```python
from build123d import *

# Parameters (mm, degrees)
SKETCH1_W                                       = 40
SKETCH1_H                                       = 20
BOSS_EXTRUDE1_DEPTH                             = 35
SKETCH2_W                                       = 5
SKETCH2_H                                       = 20
BOSS_EXTRUDE2_DEPTH                             = 5
SKETCH3_R                                       = 3.75
BOSS_EXTRUDE3_DEPTH                             = 10
CSK_FOR_M2_FLAT_HEAD_MACHINE_SCREW2_D           = 2.4
CSK_FOR_M2_FLAT_HEAD_MACHINE_SCREW2_CSINK_D     = 4.4
CSK_FOR_M2_FLAT_HEAD_MACHINE_SCREW2_CSINK_ANGLE = 90


with BuildPart() as part:
    # Sketch1 → Boss-Extrude1 (new body)
    with BuildSketch(Plane(origin=(0, 0, 0), x_dir=(1, 0, 0), z_dir=(0, 1, 0))):
        Rectangle(SKETCH1_W, SKETCH1_H)
    extrude(amount=BOSS_EXTRUDE1_DEPTH)

    # Sketch2 → Boss-Extrude2 (add)
    with BuildSketch(Plane(origin=(0, 35, 0), x_dir=(1, 0, 0), z_dir=(0, 1, 0))):
        with Locations((-22.5, 0)):
            Rectangle(SKETCH2_W, SKETCH2_H)
        with Locations((22.5, 0)):
            Rectangle(SKETCH2_W, SKETCH2_H)
    extrude(amount=-BOSS_EXTRUDE2_DEPTH)

    # Sketch3 → Boss-Extrude3 (add)
    with BuildSketch(Plane(origin=(0, 35, 0), x_dir=(1, 0, 0), z_dir=(0, 1, 0))):
        with Locations(Location((-10, 0, 0), (0, 0, 270))):
            Circle(SKETCH3_R)
    extrude(amount=BOSS_EXTRUDE3_DEPTH)

    # CSK for M2 Flat Head Machine Screw2 (through all)
    with Locations(Plane(origin=(0, 35, 0), x_dir=(1, 0, 0), z_dir=(0, 1, 0))):
        with Locations((22.5, -5), (22.5, 5)):
            csk_for_m2_flat_head_machine_screw2 = CounterSinkHole(CSK_FOR_M2_FLAT_HEAD_MACHINE_SCREW2_D / 2, CSK_FOR_M2_FLAT_HEAD_MACHINE_SCREW2_CSINK_D / 2, counter_sink_angle=CSK_FOR_M2_FLAT_HEAD_MACHINE_SCREW2_CSINK_ANGLE)

    # Mirror1: CSK for M2 Flat Head Machine Screw2 across plane
    add(csk_for_m2_flat_head_machine_screw2.mirror(Plane(origin=(0, 0, 0), x_dir=(0, 0, 1), z_dir=(1, 0, 0))), mode=Mode.SUBTRACT)


solid = part.part
```
Source: CAD feature listing. Evaluate the final solid. Frame: model axes, mm. A direction names the side the tool comes from. Coordinates: 2 decimals unless noted, no trailing zeros. Write each loop counter-clockwise with the first axis right and the second up, starting at its lowest first coordinate (ties: lowest second). Pieces come first, ordered by that corner, then holes. Notation, with made-up numbers: (-38, 86.5) -> (19, 86.5) arc R9 ccw to (19, 95.5) -> close; hole circle Ø5 at (-11.5, 86.25). An arc over 180 degrees is marked (long way). Return JSON: item names as keys, results as strings. Group by question number.
1) Section query B-B, the plane x = -22.5. Return loops of the section in (y, z), plus the area to 3 significant figures.
2) Section query C-C, the plane y = 31. Return loops of the section in (x, z).
3) Ray query, line 1 along Z through (x, y) = (22.5, 31.05); line 2 along Y through (x, z) = (22, 9.25); line 3 along Y through (x, z) = (-16, 6.5). Return the intervals inside material, ascending.
4) Section query D-D, the plane x = -10. Return loops of the section in (y, z), plus the area to 3 significant figures.
5) Set-up query: faces 4 (the face through (20, 15, 0)), 5 (the face through (0, 18, 10)), 6 (the face through (-20, 15, 0)). Return all of +Z, -Z, +X, -X, +Y, -Y with unobstructed straight access to the full face (end or side cutting, diameter ignored); none if empty.
6) Section query A-A, the plane z = -5. Return loops of the section in (x, y), plus the area to 3 significant figures.
7) Mould query, pull axis X, two halves, no side actions, for faces 1 (the face through (-6.282, 39.93, -0.488)), 2 (the face through (0, 0, 0)), 3 (the face through (23.7, 31.97, 4.95)). Classes: +X half, -X half, draft (parallel to the pull), parting line (faces both ways), or undercut.
8) Contact query for flat-ended pins moving along their axis: P1, Ø3, axis at x = 22.5, z = -5, coming from the -Y side; P2, Ø1.4, axis at x = -22.5, z = 5, coming from the +Y side; P3, Ø4, axis at x = 22.5, z = 5, coming from the +Y side; P4, Ø1.5, axis at x = -4, z = 6, coming from the +Y side. Output: stop coordinate, or through.
From the geometry:
{
 "1": {"outline": "(30, -10) -> (35, -10) -> (35, -7.2) -> (34, -6.2) -> (30, -6.2) -> close; (30, -3.8) -> (34, -3.8) -> (35, -2.8) -> (35, 2.8) -> (34, 3.8) -> (30, 3.8) -> close; (30, 6.2) -> (34, 6.2) -> (35, 7.2) -> (35, 10) -> (30, 10) -> close", "area": "74.0 mm²"},
 "2": {"outline": "(-25, -10) -> (25, -10) -> (25, 10) -> (-25, 10) -> close; hole circle Ø2.4 at (-22.5, -5); hole circle Ø2.4 at (-22.5, 5); hole circle Ø2.4 at (22.5, -5); hole circle Ø2.4 at (22.5, 5)"},
 "3": {"line 1": "-10 to -6.2, -3.8 to 3.8, 6.2 to 10", "line 2": "30 to 35", "line 3": "0 to 35"},
 "4": {"outline": "(0, -10) -> (35, -10) -> (35, -3.75) -> (45, -3.75) -> (45, 3.75) -> (35, 3.75) -> (35, 10) -> (0, 10) -> close", "area": "775 mm²"},
 "5": {"face 4": "+Z, -Z, +X, -Y", "face 5": "+Z, +X, -X, +Y, -Y", "face 6": "+Z, -Z, -X, -Y"},
 "6": {"outline": "(-25, 30) -> (-23.7, 30) -> (-23.7, 34) -> (-24.7, 35) -> (-25, 35) -> close; (-21.3, 30) -> (-20, 30) -> (-20, 0) -> (20, 0) -> (20, 30) -> (21.3, 30) -> (21.3, 34) -> (20.3, 35) -> (-20.3, 35) -> (-21.3, 34) -> close; (23.7, 30) -> (25, 30) -> (25, 35) -> (24.7, 35) -> (23.7, 34) -> close", "area": "1,420 mm²"},
 "7": {"face 1": "parting line", "face 2": "draft", "face 3": "undercut"},
 "8": {"P1": "y = 30", "P2": "through", "P3": "y = 34.8", "P4": "y = 35"}
}
